For this review, take the finished solid that the model builds, in its own axes (mm). A direction names the side the tool comes from. Round coordinates to 2 decimals unless told otherwise and drop trailing zeros. Write each loop counter-clockwise with the first axis right and the second up, starting at its lowest first coordinate (ties: lowest second). Pieces come first, ordered by that corner, then holes. Notation, with made-up numbers: M 84,8 L 119,8 A20 cw 119,36 Z; hole C 53.25,47.5 d7. An arc over 180 degrees is marked long. Answer in a Markdown table with one row per item.
```python
from build123d import *

# Parameters (mm, degrees)
SKIZZE1_R                       = 1.65
SKIZZE1_R_2                     = 4.5
SKIZZE1_W                       = 7
SKIZZE1_H                       = 0.8
AUFSATZ_LINEAR_AUSTRAGEN1_DEPTH = 12
SCHNITT_LINEAR_AUSTRAGEN2_DEPTH = 47.258945081
SCHNITT_LINEAR_AUSTRAGEN4_DEPTH = 5
VERRUNDUNG1_R                   = 10
VERRUNDUNG3_R                   = 6


with BuildPart() as part:
    # Skizze1 → Aufsatz-Linear austragen1 (new body)
    with BuildSketch(Plane(origin=(0, 0, 0), x_dir=(0, 0, -1), z_dir=(1, 0, 0))):
        with BuildLine():
            Line((13.995498987, 0), (23, 0))
            Line((23, 0), (23, 38.3))
            Line((23, 38.3), (0, 38.3))
            Line((0, 38.3), (0, 9.46515139))
            ThreePointArc((0, 9.46515139), (-1.602122342, -7.983491128), (13.995498987, 0))
        make_face()
        with Locations((4, 33.8)):
            Circle(SKIZZE1_R, mode=Mode.SUBTRACT)
        with Locations((19, 33.8)):
            Circle(SKIZZE1_R, mode=Mode.SUBTRACT)
        with Locations((4, 0.3)):
            Circle(SKIZZE1_R_2, mode=Mode.SUBTRACT)
        with Locations((16.5, 3.4)):
            Rectangle(SKIZZE1_W, SKIZZE1_H, mode=Mode.SUBTRACT)
        with Locations((16.5, 7.2)):
            Rectangle(SKIZZE1_W, SKIZZE1_H, mode=Mode.SUBTRACT)
        with Locations((16.5, 11)):
            Rectangle(SKIZZE1_W, SKIZZE1_H, mode=Mode.SUBTRACT)
    extrude(amount=AUFSATZ_LINEAR_AUSTRAGEN1_DEPTH)

    # Skizze2 → Schnitt-Linear austragen2 (cut, through all)
    with BuildSketch(Plane.XY):
        with BuildLine():
            Line((3.5, 38.3), (8.5, 38.3))
            Line((8.5, 38.3), (8.5, 27.458312395))
            ThreePointArc((8.5, 27.458312395), (6, 22.8), (3.5, 27.458312395))
            Line((3.5, 27.458312395), (3.5, 38.3))
        make_face()
    extrude(amount=-SCHNITT_LINEAR_AUSTRAGEN2_DEPTH, mode=Mode.SUBTRACT)

    # Skizze5 → Schnitt-Linear austragen4 (cut)
    with BuildSketch(Plane(origin=(0, 0, 0), x_dir=(0, 0, -1), z_dir=(1, 0, 0))):
        Polygon((0.102885683, 7.05), (-3.794228634, 0.3), (0.102885683, -6.45), (7.897114317, -6.45), (11.794228634, 0.3), (7.897114317, 7.05), align=None)
    extrude(amount=SCHNITT_LINEAR_AUSTRAGEN4_DEPTH, mode=Mode.SUBTRACT)

    # Verrundung1
    verrundung1_edges = [part.edges().sort_by_distance(p)[0] for p in [
        (6, 0, -13.995498987),
        (6, 9.46515139, 0),
    ]]
    fillet(verrundung1_edges, radius=VERRUNDUNG1_R)

    # Verrundung3
    verrundung3_edges = [part.edges().sort_by_distance(p)[0] for p in [
        (6, 0, -23),
    ]]
    fillet(verrundung3_edges, radius=VERRUNDUNG3_R)


solid = part.part
```
Q1. For probe 1 along Z at (x, y) = (2, 33.8); probe 2 along X at (y, z) = (35.5, -21); probe 3 along Y at (x, z) = (1.75, -16), list the stretches that pass through material, from the lowest coordinate up.
Found:
| item | result |
|---|---|
| probe 1 | -23 to -20.65, -17.35 to -5.65, -2.35 to 0 |
| probe 2 | 0 to 3.5, 8.5 to 12 |
| probe 3 | -1.42 to 3, 3.8 to 6.8, 7.6 to 10.6, 11.4 to 38.3 |
Q2. Take a section at C-C (y = 25.8). State the section outline as (x, z) points.
Found:
| item | result |
|---|---|
| outline | M 0,-23 L 3,-23 L 3,0 L 0,0 Z; M 9,-23 L 12,-23 L 12,0 L 9,0 Z |
Q3. Take a section at A-A (y = 33.8). State the section outline as (x, z) points.
Found:
| item | result |
|---|---|
| outline | M 0,-23 L 3.5,-23 L 3.5,-20.65 L 0,-20.65 Z; M 0,-17.35 L 3.5,-17.35 L 3.5,-5.65 L 0,-5.65 Z; M 0,-2.35 L 3.5,-2.35 L 3.5,0 L 0,0 Z; M 8.5,-23 L 12,-23 L 12,-20.65 L 8.5,-20.65 Z; M 8.5,-17.35 L 12,-17.35 L 12,-5.65 L 8.5,-5.65 Z; M 8.5,-2.35 L 12,-2.35 L 12,0 L 8.5,0 Z |
Q4. Insertion check: P1, Ø1.5, axis at x = 8.5, z = 1, coming from the -Y side; P2, Ø2, axis at x = 4, z = -17.5, coming from the -Y side; P3, Ø6, axis at x = 1, y = 13, coming from the +Z side; P4, Ø5.5, axis at y = 0.3, z = -4, coming from the +X side (3 decimals). Each pin has a flat end and moves straight along its axis. Give the tip position at first contact, or say it passes through.
Found:
| item | result |
|---|---|
| P1 | y = -8.75 |
| P2 | y = -1.14 |
| P3 | z = 1.11 |
| P4 | through |
Q5. Machinability: for faces 1 (the face through (2, 7.05, -4)), 2 (the face through (6, 11.4, -16)), 3 (the face through (10, 38.3, -12)), which of the approach directions +Z, -Z, +X, -X, +Y, -Y give a long, thin tool a straight path to every point of the face, cutting with its end or side? Answer none if there is none.
Found:
| item | result |
|---|---|
| face 1 | -X |
| face 2 | +X, -X |
| face 3 | +Z, -Z, +X, -X, +Y |
Q6. Take a section at D-D (x = 6). State how many separate pieces and enclosed holes the cut face has, then the cut area to 3 significant figures.
Found:
| item | result |
|---|---|
| separate pieces | 1 |
| enclosed holes | 4 |
| area | 642 mm² |
Q7. Take a section at B-B (z = -14.75). State the section outline as (x, y) points, then the cut area to 3 significant figures.
Found:
| item | result |
|---|---|
| outline | M 0,-2.31 L 12,-2.31 L 12,3 L 0,3 Z; M 0,3.8 L 12,3.8 L 12,6.8 L 0,6.8 Z; M 0,7.6 L 12,7.6 L 12,10.6 L 0,10.6 Z; M 0,11.4 L 12,11.4 L 12,38.3 L 8.5,38.3 L 8.5,27.46 A3 cw long 3.5,27.46 L 3.5,38.3 L 0,38.3 Z |
| area | 381 mm² |
Q8. Mouldability with a two-part tool opening along X and no side actions: class faces 4 (the face through (8.5, 33, -11)), 5 (the face through (3.5, 33, -11)), 6 (the face through (6, 6.8, -16)), 7 (the face through (0, 15, -12)) as +X half, -X half, draft (parallel to the pull), parting line (faces both ways), or undercut.
Found:
| item | result |
|---|---|
| face 4 | undercut |
| face 5 | undercut |
| face 6 | draft |
| face 7 | -X half |
